from build123d import *

# Parameters (mm, degrees)
SZKIC1_R                    = 31
DODANIE_WYCI_GNI_CIE1_DEPTH = 4
DODANIE_WYCI_GNI_CIE2_DEPTH = 6
SZKIC3_R                    = 1.2
WYTNIJ_WYCI_GNI_CIE1_DEPTH  = 51.813384064
SZYK_KO_OWY1_COUNT          = 3
SZKIC4_R                    = 1.6
WYTNIJ_WYCI_GNI_CIE2_DEPTH  = 6
WYTNIJ_WYCI_GNI_CIE3_DEPTH  = 45.24929378


with BuildPart() as part:
    # Szkic1 → Dodanie-wyciągnięcie1 (new body)
    with BuildSketch(Plane.XY):
        Circle(SZKIC1_R)
    extrude(amount=DODANIE_WYCI_GNI_CIE1_DEPTH)

    # Szkic2 → Dodanie-wyciągnięcie2 (add)
    with BuildSketch(Plane.XY.offset(4)):
        Polygon((4.618802154, 8), (-4.618802154, 8), (-9.237604307, 0), (-4.618802154, -8), (4.618802154, -8), (9.237604307, 0), align=None)
        Polygon((1.962990915, 3.4), (-1.962990915, 3.4), (-3.92598183, 0), (-1.962990915, -3.4), (1.962990915, -3.4), (3.92598183, 0), align=None, mode=Mode.SUBTRACT)
    extrude(amount=DODANIE_WYCI_GNI_CIE2_DEPTH)

    # Szkic3 → Wytnij-wyciągnięcie1 (cut, through all)
    with BuildSketch(Plane(origin=(0, 8, 0), x_dir=(1, 0, 0), z_dir=(0, 1, 0))):
        with Locations(Location((0, -7, 0), (0, 0, 180))):
            Circle(SZKIC3_R)
    wytnij_wyci_gni_cie1 = extrude(amount=-WYTNIJ_WYCI_GNI_CIE1_DEPTH, mode=Mode.SUBTRACT)

    # Szyk kołowy1: Wytnij-wyciągnięcie1 ×3 about axis
    szyk_ko_owy1_axis = Axis((0, 0, 4), (0, 0, 1))
    for i in range(1, SZYK_KO_OWY1_COUNT):
        add(wytnij_wyci_gni_cie1.rotate(szyk_ko_owy1_axis, i * 360 / SZYK_KO_OWY1_COUNT), mode=Mode.SUBTRACT)

    # Szkic4 → Wytnij-wyciągnięcie2 (cut)
    with BuildSketch(Plane.XY.offset(4)):
        with Locations((0, 17.5)):
            Circle(SZKIC4_R)
        with Locations((17.5, 0)):
            Circle(SZKIC4_R)
        with Locations((0, -17.5)):
            Circle(SZKIC4_R)
        with Locations((-17.5, 0)):
            Circle(SZKIC4_R)
    extrude(amount=-WYTNIJ_WYCI_GNI_CIE2_DEPTH, mode=Mode.SUBTRACT)

    # Szkic5 → Wytnij-wyciągnięcie3 (cut, through all)
    with BuildSketch(Plane.XY.offset(4)):
        Polygon((3.92598183, 0), (1.962990915, 3.4), (-1.962990915, 3.4), (-3.92598183, 0), (-1.962990915, -3.4), (1.962990915, -3.4), align=None)
    extrude(amount=-WYTNIJ_WYCI_GNI_CIE3_DEPTH, mode=Mode.SUBTRACT)


solid = part.part
Can you work these out from the model? Positions are in its coordinate system, mm. A direction names the side the tool comes from. Give positions to 0.01 mm unless a question says otherwise; leave off trailing zeros. Loops run counter-clockwise (first coordinate to the right, second up) from the corner with the lowest first, then second, coordinate; pieces in that order, holes last. Notation, with made-up numbers: (7.25, -23.75) -> (15.25, -23.75) arc R24 cw to (15.25, 6.25) -> close; hole circle Ø8 at (-15.5, 32). An arc over 180 degrees is marked (long way). Write item = value, one per line.
1) Will these pins go through, and if not, where does the flat tip stop? pin 1 (3.5 mm diameter, centred on x = -17.5, y = 0, fed in from +Z); pin 2 (2 mm diameter, centred on x = -14.5, z = 3, fed in from +Y); pin 3 (3 mm diameter, centred on x = -2.5, z = 7, fed in from +Y).
Check result:
pin_1 = 4
pin_2 = 27.91
pin_3 = 8
2) Suppose I cut it at B-B on z = 2.75. Write out the boundary of the cut face in (x, y).
Check result:
outline = circle Ø62 at (0, 0); hole circle Ø3.2 at (-17.5, 0); hole (-3.93, 0) -> (-1.96, -3.4) -> (1.96, -3.4) -> (3.93, 0) -> (1.96, 3.4) -> (-1.96, 3.4) -> close; hole circle Ø3.2 at (0, -17.5); hole circle Ø3.2 at (0, 17.5); hole circle Ø3.2 at (17.5, 0)
3) Suppose I cut it at C-C on y = -17.5. Write out the boundary of the cut face in (x, z), then the cut area to 3 significant figures.
Check result:
outline = (-25.59, 0) -> (-1.6, 0) -> (-1.6, 4) -> (-25.59, 4) -> close; (1.6, 0) -> (25.59, 0) -> (25.59, 4) -> (1.6, 4) -> close
area = 192 mm2
4) I need wall thicknesses on L1, parallel to Y at x = 0, z = 1.9; L2, parallel to Z at x = 0, y = -5; L3, parallel to Z at x = -24, y = 5. Which ranges of each line are inside material? Lowest first, please. Write a range as from..to.
Check result:
L1 = -31..-19.1, -15.9..-3.4, 3.4..15.9, 19.1..31
L2 = 0..5.8, 8.2..10
L3 = 0..4
5) For faces 4 (the flat face through (6.961, 3.944, 5.625)), 5 (the flat face through (0, -3.4, 5)), 6 (the flat face through (1, 8, 8)), 7 (the flat face through (-1, -8, 8)), 8 (the flat face through (-6.896, 4.056, 5.625)), which set-ups out of +Z, -Z, +X, -X, +Y, -Y let a thin tool reach every point of the face, with its end or its side?
Check result:
face_4 = +Z, +X, +Y
face_5 = +Z, -Z
face_6 = +Z, +X, -X, +Y
face_7 = +Z, +X, -X, -Y
face_8 = +Z, -X, +Y
6) Thinking about a two-plate mould opening in Z: for faces 1 (the cylindrical face through (0.16, 5.73, 8.19)), 2 (the flat face through (0, 4, 10)), 3 (the flat face through (-6.961, -3.944, 5.625)), which applies, released by +Z, released by -Z, zero draft, split by the parting line, or undercut?
Check result:
face_1 = undercut
face_2 = released by +Z
face_3 = zero draft
7) Suppose I cut it at A-A on x = 0. Write out the boundary of the cut face in (y, z), then the cut area to 3 significant figures.
Check result:
outline = (-31, 0) -> (-19.1, 0) -> (-19.1, 4) -> (-31, 4) -> close; (-15.9, 0) -> (-3.4, 0) -> (-3.4, 5.8) -> (-8, 5.8) -> (-8, 4) -> (-15.9, 4) -> close; (-8, 8.2) -> (-3.4, 8.2) -> (-3.4, 10) -> (-8, 10) -> close; (3.4, 0) -> (15.9, 0) -> (15.9, 4) -> (8, 4) -> (8, 5.8) -> (3.4, 5.8) -> close; (3.4, 8.2) -> (8, 8.2) -> (8, 10) -> (3.4, 10) -> close; (19.1, 0) -> (31, 0) -> (31, 4) -> (19.1, 4) -> close
area = 228 mm2
